Input: part model. Units: mm. Frame: model coordinates. A direction names the side the tool comes from. Coordinates: 2 decimals unless noted, no trailing zeros. Order: outer loops, then holes, each group sorted by start corner. A loop starts at its lowest first (then second) coordinate and runs counter-clockwise, first axis right, second up. Notation, with made-up numbers: (28, 52) - (50, 52) arc R30 cw to (50, 91) - close; hole circle Ø8 at (6.5, -3). An arc over 180 degrees is marked (long way). Answer as CSV lines item,"result". Start each with the question number.
Item 1: Section D-D (z = 12.75). Output: boundary loops of the cut face in (x, y).
Item 2: Material intervals for line 1 along X through (y, z) = (36, 3.25); line 2 along X through (y, z) = (30, 16); line 3 along X through (y, z) = (31, 11.5), sorted ascending.
Item 3: First-contact query: pin 1 (17 mm diameter, centred on x = 36.5, y = 35, fed in from +Z); pin 2 (6 mm diameter, centred on x = 13, y = 33.5, fed in from +Z). Flat tips, straight axial feed; report the tip coordinate or a pass-through.
Item 4: Access query for faces 4 (the flat face through (34, 0, 10)), 5 (the flat face through (6.35, 38, 9)). Directions: +Z, -Z, +X, -X, +Y, -Y. A direction counts if a zero-diameter tool reaches every point of the face in a straight line with its end or side. Return the directions, or none.
Item 5: Section C-C (x = 48). Output: boundary loops of the cut face in (y, z), and give its area (3 significant figures).
Item 6: Section A-A (z = 5.5). Output: boundary loops of the cut face in (x, y), and give its area (3 significant figures).
Item 7: Draft query along X for faces 1 (the flat face through (26.67, 34, 2)), 2 (the flat face through (35, 46.228, 10)), 3 (the cylindrical face through (67.82, 45.5, 9.52)). Return one class per face: +X half, -X half, draft (parallel to the pull), parting line (faces both ways), or undercut.
Item 8: Section B-B (x = 34.29). Output: boundary loops of the cut face in (y, z), and give its area (3 significant figures).
Autodesk Inventor part; units mm, degrees
ref_plane "YZ Plane" through (0, 0, 0) normal (1, 0, 0) x (0, 1, 0)
ref_plane "XZ Plane" through (0, 0, 0) normal (0, 1, 0) x (-1, 0, 0)
ref_plane "XY Plane" through (0, 0, 0) normal (0, 0, 1) x (1, 0, 0)
sketch "Sketch1" plane through (0, 0, 0) normal (0, 0, 1) x (1, 0, 0)
  line L0 (0, 0) -> (68.58, 0)
  line L1 (68.58, 0) -> (68.58, 46.228)
  line L2 (68.58, 46.228) -> (0, 46.228)
  line L3 (0, 46.228) -> (0, 0)
  dimension "d0" = 68.58
  dimension "d1" = 46.228
extrude "Extrusion1" add sketch "Sketch1" along normal blind 2.54
sketch "Sketch2" plane through (0, 0, 2.54) normal (0, 0, 1) x (1, 0, 0)
  line L0 (0, 46.228) -> (0, 0)
  line L1 (0, 46.228) -> (68.58, 46.228)
  line L2 (68.58, 46.228) -> (68.58, 0)
  line L3 (68.58, 0) -> (0, 0)
  line L4 (0, 0) -> (0, 46.228)
  line L5 (6.35, 43.688) -> (59.69, 43.688)
  line L6 (59.69, 43.688) -> (59.69, 28.448)
  line L7 (59.69, 28.448) -> (6.35, 28.448)
  line L8 (6.35, 28.448) -> (6.35, 43.688)
  line L9 (3.048, 28.448) -> (65.532, 28.448)
  line L10 (65.532, 28.448) -> (65.532, 3.048)
  line L11 (65.532, 3.048) -> (3.048, 3.048)
  line L12 (3.048, 3.048) -> (3.048, 28.448)
  dimension "d4" = 62.484
  dimension "d5" = 53.34
  dimension "d6" = 15.24
  dimension "d7" = 25.4
  dimension "d8" = 3.048
  dimension "d9" = 3.048
  dimension "d10" = 0
  dimension "d13" = 6.35
extrude "Extrusion2" add sketch "Sketch2" along normal blind 16.764
chamfer "Chamfer1" distance 6.35 distance2 12.7 1 edges at (62.611, 28.448, 19.304) measured on face at (23.876, 1.016, 19.304)
chamfer "Chamfer2" distance 6.35 distance2 12.7 1 edges at (4.699, 28.448, 19.304) measured on face at (23.876, 1.016, 19.304)
sketch "Sketch3" plane through (0, 0, 2.54) normal (0, 0, 1) x (1, 0, 0)
  circle A0 centre (34.29, 36.068) radius 3.4925
  line L0 (0, 0) -> (68.58, 0)
  line L1 (0, 46.228) -> (0, 0)
  line L2 (68.58, 46.228) -> (0, 46.228)
  line L3 (68.58, 0) -> (68.58, 46.228)
  dimension "d22" = 10.16
  dimension "d23" = 34.29
  dimension "d24" = 6.985
extrude "Extrusion3" cut sketch "Sketch3" against normal up to surface (2.54 mm away) contours A0
sketch "Sketch4" plane through (0, 0, 2.54) normal (0, 0, 1) x (1, 0, 0)
  line L0 (59.69, 28.448) -> (59.69, 43.688)
  line L1 (59.69, 43.688) -> (6.35, 43.688)
  circle A0 centre (44.704, 36.068) radius 1.4732
  point P0 (0, 0)
  dimension "d27" = 2.9464
  dimension "d28" = 7.62
  dimension "d29" = 14.986
extrude "Extrusion4" add sketch "Sketch4" along normal blind 7.62
fillet "Fillet1" radius 1.4732 1 edges at (43.2308, 36.068, 10.16)
fillet "Fillet2" radius 2.54 2 edges at (0, 46.228, 9.652) (68.58, 46.228, 9.652)
sketch "Sketch5" plane through (0, 0, 2.54) normal (0, 0, 1) x (1, 0, 0)
  circle A0 centre (34.29, 36.068) radius 3.4925
  line L0 (26.67, 43.688) -> (41.91, 43.688)
  line L1 (41.91, 43.688) -> (41.91, 24.638)
  line L2 (41.91, 24.638) -> (26.67, 24.638)
  line L3 (26.67, 24.638) -> (26.67, 43.688)
  point P0 (0, 0)
  dimension "d34" = 19.05
  dimension "d35" = 15.24
  dimension "d36" = 7.62
  dimension "d37" = 7.62
extrude "Extrusion5" cut sketch "Sketch5" against normal blind 1.524
hole "Hole1" at (68.58, 37.338, 12.954) direction (-1, 0, 0) diameter 4.1656 end through all
equation "\"d9\" = d8"
properties part number "Case_Cutout"
Determined:
1,outline,"(0, 0) - (68.58, 0) - (68.58, 35.27) - (59.69, 35.27) - (59.69, 31.52) - (65.53, 31.52) - (65.53, 3.05) - (3.05, 3.05) - (3.05, 31.52) - (6.35, 31.52) - (6.35, 35.27) - (0, 35.27) - close; (0, 39.41) - (6.35, 39.41) - (6.35, 43.69) - (59.69, 43.69) - (59.69, 39.41) - (68.58, 39.41) - (68.58, 43.69) arc R2.54 ccw to (66.04, 46.23) - (2.54, 46.23) arc R2.54 ccw to (0, 43.69) - close"
2,line 1,"x = 0 to 6.35, 43.23 to 46.18, 59.69 to 68.58"
2,line 2,"x = 0 to 3.05, 65.53 to 68.58"
2,line 3,"x = 0 to 6.35, 59.69 to 68.58"
3,pin 1,"stops at z = 10.16"
3,pin 2,"stops at z = 2.54"
4,face 4,"+Z, -Z, +X, -X, -Y"
4,face 5,"+Z"
5,outline,"(0, 0) - (46.23, 0) - (46.23, 19.3) - (43.69, 19.3) - (43.69, 2.54) - (3.05, 2.54) - (3.05, 19.3) - (0, 19.3) - close"
5,area,"211 mm^2"
6,outline,"(0, 0) - (68.58, 0) - (68.58, 43.69) arc R2.54 ccw to (66.04, 46.23) - (2.54, 46.23) arc R2.54 ccw to (0, 43.69) - close; circle Ø2.95 at (44.7, 36.07); hole (3.05, 3.05) - (65.53, 3.05) - (65.53, 28.45) - (59.69, 28.45) - (59.69, 43.69) - (6.35, 43.69) - (6.35, 28.45) - (3.05, 28.45) - close"
6,area,"774 mm^2"
7,face 1,"undercut"
7,face 2,"draft"
7,face 3,"+X half"
8,outline,"(0, 0) - (32.58, 0) - (32.58, 1.02) - (24.64, 1.02) - (24.64, 2.54) - (3.05, 2.54) - (3.05, 19.3) - (0, 19.3) - close; (39.56, 0) - (46.23, 0) - (46.23, 19.3) - (43.69, 19.3) - (43.69, 1.02) - (39.56, 1.02) - close"
8,area,"175 mm^2"
